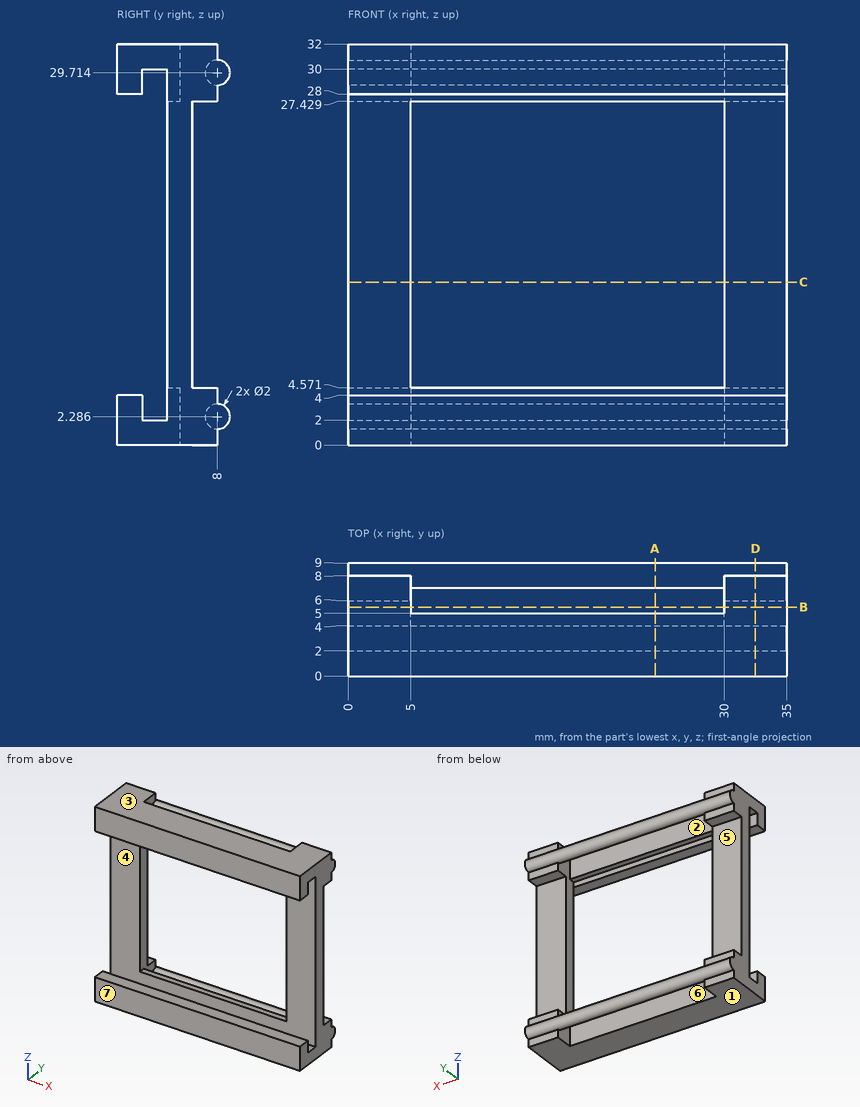
Print and shaded views of the part. All mm, measured from the part's lowest x, y and z. A direction names the side the tool comes from. Coordinates: 2 decimals unless noted, no trailing zeros. Loops run counter-clockwise (first coordinate to the right, second up) from the corner with the lowest first, then second, coordinate; pieces in that order, holes last. Notation, with made-up numbers: (39.5, 12.5) -> (87.5, 12.5) arc R18 cw to (87.5, 29.5) -> close; hole circle Ø9 at (-26.5, 26). An arc over 180 degrees is marked (long way). Use a Markdown table: item, result. Add a question column.
Item 1: Which spindle directions (+Z, -Z, +X, -X, +Y, -Y) get a long thin tool onto all of the face, cutting with end or side? Do the marked faces 5, 6 and 7. Say none if no direction does.
Item 2: Band-saw the part on C-C on z = 13. Write the cut outline in (x, y), plus the area to 3 significant figures.
Item 3: Band-saw the part on A-A on x = 24.5. Write the cut outline in (y, z) (1 decimal).
Item 4: Probe probe 1 along X at (y, z) = (5.5, 10); probe 2 along Y at (x, z) = (18.5, 3); probe 3 along Z at (x, y) = (27.5, 4.75). List the from-to ranges inside material, lowest first.
Item 5: Band-saw the part on D-D on x = 32.5. Write the cut outline in (y, z) (1 decimal).
Item 6: Pull direction Z, two halves, no side cores. Call the marked faces 1, 2, 3 and 4: +Z half, -Z half, draft (parallel to the pull), parting line (faces both ways), or undercut.
Item 7: Flat gauge pins, fed straight in: P1, Ø1, axis at x = 1.5, z = 28, coming from the +Y side; P2, Ø12, axis at x = 13.5, z = 20, coming from the -Y side (3 decimals). Where does each tip first touch, or does it go through?
Item 8: Band-saw the part on B-B on y = 5.5. Write the cut outline in (x, z).
Geometry says:
| question | item | result |
|---|---|---|
| 1 | face 5 | +X, -X, +Y |
| 1 | face 6 | +Z, -Z |
| 1 | face 7 | +Z, -Z, +X, -X, -Y |
| 2 | outline | (0, 4) -> (5, 4) -> (5, 6) -> (0, 6) -> close; (30, 4) -> (35, 4) -> (35, 6) -> (30, 6) -> close |
| 2 | area | 20.0 mm² |
| 3 | outline | (0, 0) -> (5, 0) -> (5, 4.6) -> (4, 4.6) -> (4, 2) -> (2, 2) -> (2, 4) -> (0, 4) -> close; (0, 28) -> (2, 28) -> (2, 30) -> (4, 30) -> (4, 27.4) -> (5, 27.4) -> (5, 32) -> (0, 32) -> close; circle Ø2 at (8, 2.3); circle Ø2 at (8, 29.7) |
| 4 | probe 1 | 0 to 5, 30 to 35 |
| 4 | probe 2 | 0 to 2, 4 to 5, 7.3 to 8.7 |
| 4 | probe 3 | 0 to 4.57, 27.43 to 32 |
| 5 | outline | (0, 0) -> (8, 0) -> (8, 1.3) arc R1 ccw to (8, 3.3) -> (8, 4.6) -> (6, 4.6) -> (6, 27.4) -> (8, 27.4) -> (8, 28.7) arc R1 ccw to (8, 30.7) -> (8, 32) -> (0, 32) -> (0, 28) -> (2, 28) -> (2, 30) -> (4, 30) -> (4, 2) -> (2, 2) -> (2, 4) -> (0, 4) -> close |
| 6 | face 1 | -Z half |
| 6 | face 2 | draft |
| 6 | face 3 | +Z half |
| 6 | face 4 | undercut |
| 7 | P1 | y = 8 |
| 7 | P2 | through |
| 8 | outline | (0, 0) -> (5, 0) -> (5, 32) -> (0, 32) -> close; (30, 0) -> (35, 0) -> (35, 32) -> (30, 32) -> close |
